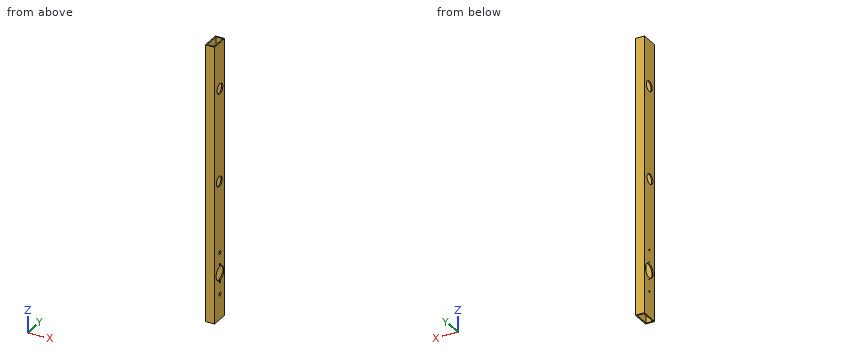
Autodesk Inventor part; units mm, degrees
ref_plane "YZ Plane" through (0, 0, 0) normal (1, 0, 0) x (0, 1, 0)
ref_plane "XZ Plane" through (0, 0, 0) normal (0, 1, 0) x (-1, 0, 0)
ref_plane "XY Plane" through (0, 0, 0) normal (0, 0, 1) x (1, 0, 0)
sketch "Sketch1" plane through (0, 0, 0) normal (0, 1, 0) x (-1, 0, 0)
  point P0 (0, 0)
sketch "Sketch2" plane through (0, 0, 0) normal (0, 1, 0) x (-1, 0, 0)
  line L0 (0, 0) -> (25.4, 0)
  line L1 (25.4, 0) -> (25.4, -812.8)
  line L2 (25.4, -812.8) -> (0, -812.8)
  line L3 (0, -812.8) -> (0, 0)
  dimension "d0" = 812.8
  dimension "d1" = 25.4
extrude "Extrusion1" add sketch "Sketch2" along normal blind 50.8
sketch "Sketch3" plane through (0, 0, 0) normal (1, 0, 0) x (0, 0, -1)
  circle A0 centre (152.4, 26.9875) radius 14.2875
  line L0 (0, 0) -> (0, 50.8)
  line L1 (0, 50.8) -> (812.8, 50.8)
  circle A1 centre (660.4, 26.9875) radius 19.05
  line L2 (812.8, 0) -> (812.8, 50.8)
  line L3 (812.8, 0) -> (0, 0)
  circle A2 centre (406.4, 23.8125) radius 14.2875
  point P0 (406.4, 50.8)
  point P1 (406.4, 0)
  point P2 (406.4, 0)
  dimension "d4" = 28.575
  dimension "d5" = 152.4
  dimension "d6" = 23.8125
  dimension "d7" = 38.1
  dimension "d8" = 152.4
  dimension "d9" = 26.9875
  dimension "d10" = 28.575
  dimension "d11" = 26.9875
extrude "Extrusion2" cut sketch "Sketch3" against normal through all contours A0 | A1 | A2
sketch "Sketch4" plane through (-25.4, 0, 0) normal (0, 0, 1) x (1, 0, 0)
  line L0 (0, 50.8) -> (25.4, 50.8)
  line L1 (25.4, 0) -> (25.4, 50.8)
  line L2 (25.4, 0) -> (0, 0)
  line L3 (0, 0) -> (0, 50.8)
  line L4 (22.225, 47.625) -> (3.175, 47.625)
  line L5 (3.175, 47.625) -> (3.175, 3.175)
  line L6 (3.175, 3.175) -> (22.225, 3.175)
  line L7 (22.225, 3.175) -> (22.225, 47.625)
  dimension "d15" = 3.175
extrude "Extrusion3" cut sketch "Sketch4" against normal up to surface (812.8 mm away) contours L7 L6 L5 L4
sketch "Sketch5" plane through (0, 0, 0) normal (1, 0, 0) x (0, 0, -1)
  circle A0 centre (660.4, 26.9875) radius 19.05
  circle A1 centre (152.4, 26.9875) radius 14.2875
  circle A2 centre (406.4, 23.8125) radius 14.2875
  line L0 (812.8, 0) -> (0, 0)
  line L1 (812.8, 0) -> (812.8, 50.8)
  line L2 (0, 50.8) -> (812.8, 50.8)
  line L3 (0, 0) -> (0, 50.8)
  line L4 (0, 50.8) -> (25.4, 50.8)
  line L5 (25.4, 50.8) -> (25.4, 0)
  line L6 (25.4, 0) -> (0, 0)
  line L7 (0, 0) -> (0, 50.8)
  line L8 (812.8, 0) -> (812.8, 50.8)
  line L9 (812.8, 0) -> (0, 0)
  line L10 (812.8, 50.8) -> (787.4, 50.8)
  line L11 (787.4, 50.8) -> (787.4, 0)
  line L12 (787.4, 0) -> (812.8, 0)
  line L13 (812.8, 0) -> (812.8, 50.8)
  dimension "d18" = 25.4
  dimension "d19" = 25.4
  dimension "d59" = 38.1
extrude "Extrusion4" cut sketch "Sketch5" against normal blind 25.4 contours L0 L11 L2 L1 | L0 L3 L2 L5
sketch "Sketch6" plane through (0, 0, -25.4) normal (1, 0, 0) x (0, 0, -1)
  line L0 (762, 0) -> (762, 50.8)
  circle A0 centre (635, 26.9875) radius 19.05
  line L1 (0, 50.8) -> (762, 50.8)
  line L2 (0, 50.8) -> (0, 0)
  line L3 (762, 0) -> (0, 0)
  line L4 (762, 0) -> (762, 50.8)
  line L5 (0, 50.8) -> (762, 50.8)
  circle A1 centre (635, 26.9875) radius 19.05
  circle A2 centre (127, 26.9875) radius 14.2875
  circle A3 centre (381, 23.8125) radius 14.2875
  point P0 (-25.4, 0)
  point P1 (658.8125, 26.9875)
  point P2 (611.1875, 26.9875)
  point P3 (692.1754, 26.9875)
  point P4 (577.8246, 26.9875)
  dimension "d37" = 47.625
  dimension "d38" = 23.8125
  dimension "d39" = 57.1754
  dimension "d40" = 57.1754
  dimension "d60" = 38.1
hole "Hole1" at (0, 26.9875, -717.5754) at (0, 26.9875, -603.2246) direction (-1, 0, 0) diameter 4.9784 end through all counterbore diameter 9.525 counterbore depth 6.35
sketch "Sketch7" plane through (0, 0, -25.4) normal (1, 0, 0) x (0, 0, -1)
  circle A0 centre (635, 26.9875) radius 19.05
  point P0 (-25.4, 0)
  point P1 (658.8125, 26.9875)
  point P2 (611.1875, 26.9875)
  dimension "d48" = 47.625
  dimension "d49" = 23.8125
  dimension "d50" = 23.8125
  dimension "d58" = 38.1
hole "Hole2" at (0, 26.9875, -636.5875) at (0, 26.9875, -684.2125) direction (-1, 0, 0) diameter 3.175 end through all counterbore diameter 6.35 counterbore depth 6.35
equation "\"d9\" = d11"
properties part number "2x1 20in Alluminum with Cal DropRighttSide.ver1-1111-2019"
Design review of the part built by this model. Coordinates are the model's own, in mm. Round coordinates to 2 decimals unless told otherwise and drop trailing zeros. Order: outer loops, then holes, each group sorted by start corner. A loop starts at its lowest first (then second) coordinate and runs counter-clockwise, first axis right, second up.
1) Consider section D-D (z = -406.4). State the section outline as (x, y) points (3 decimals).
The answers:
outline: (-25.4, 0) - (0, 0) - (0, 9.525) - (-3.175, 9.525) - (-3.175, 3.175) - (-22.225, 3.175) - (-22.225, 9.525) - (-25.4, 9.525) - close; (-25.4, 38.1) - (-22.225, 38.1) - (-22.225, 47.625) - (-3.175, 47.625) - (-3.175, 38.1) - (0, 38.1) - (0, 50.8) - (-25.4, 50.8) - close
2) Consider section A-A (z = -660.4). State the section outline as (x, y) points (1 decimal).
The answers:
outline: (-25.4, 0) - (0, 0) - (0, 7.9) - (-3.2, 7.9) - (-3.2, 3.2) - (-22.2, 3.2) - (-22.2, 7.9) - (-25.4, 7.9) - close; (-25.4, 46) - (-22.2, 46) - (-22.2, 47.6) - (-3.2, 47.6) - (-3.2, 46) - (0, 46) - (0, 50.8) - (-25.4, 50.8) - close
3) For L1, parallel to Y at x = -13.5, z = -103 (3 decimals); L2, parallel to X at y = 9.5, z = -614.5 (3 decimals); L3, parallel to Y at x = -1.1, z = -152.4 (3 decimals), list the stretches that pass through material, from the lowest coordinate up.
The answers:
L1: y = 0 to 3.175, 47.625 to 50.8
L2: x = -25.4 to -22.225, -3.175 to 0
L3: y = 0 to 12.7, 41.275 to 50.8
4) Consider section B-B (x = -12.5). State the section outline as (y, z) points (3 decimals).
The answers:
outline: (0, -787.4) - (3.175, -787.4) - (3.175, -25.4) - (0, -25.4) - close; (47.625, -787.4) - (50.8, -787.4) - (50.8, -25.4) - (47.625, -25.4) - close
5) Consider section C-C (z = -522). State the section outline as (x, y) points (3 decimals).
The answers:
outline: (-25.4, 0) - (0, 0) - (0, 50.8) - (-25.4, 50.8) - close; hole (-22.225, 3.175) - (-3.175, 3.175) - (-3.175, 47.625) - (-22.225, 47.625) - close
6) Clearance check with flat-ended pins moving along their axes: pin 1 Ø2 at (y, z) = (15, -370.5) entering from +X; pin 2 Ø4.5 at (y, z) = (26.99, -717.58) entering from +X; pin 3 Ø5.5 at (y, z) = (26.99, -603.22) entering from +X (3 decimals). State where each tip first meets the part, or that it passes through.
The answers:
pin 1: stops at x = 0
pin 2: passes through
pin 3: stops at x = -22.225
